from build123d import *

# Parameters (mm, degrees)
SKETCH1_R           = 4.7625
BOSS_EXTRUDE1_DEPTH = 0.79375
SKETCH2_R           = 3.9751
BOSS_EXTRUDE2_DEPTH = 5.461
SKETCH3_R           = 3.3147
BOSS_EXTRUDE3_DEPTH = 12.065
SKETCH6_R           = 1.5875
CUT_EXTRUDE1_DEPTH  = 19.05
SKETCH10_W          = 1.27
SKETCH10_H          = 1.778
SKETCH11_R          = 0.0508
CUT_EXTRUDE3_DEPTH  = 0.0254
SKETCH9_R           = 0.02
CUT_EXTRUDE2_DEPTH  = 23.4028
CHAMFER1_SIZE       = 1.27


with BuildPart() as part:
    # Sketch1 → Boss-Extrude1 (new body, symmetric)
    with BuildSketch(Plane.XY):
        Circle(SKETCH1_R)
    extrude(amount=BOSS_EXTRUDE1_DEPTH, both=True)

    # Sketch2 → Boss-Extrude2 (add)
    with BuildSketch(Plane(origin=(0, 0, -0.79375), x_dir=(-1, 0, 0), z_dir=(0, 0, -1))):
        with Locations(Location((0, 0, 0), (0, 0, 180))):  # turned: the seam where the file's is
            Circle(SKETCH2_R)
    extrude(amount=BOSS_EXTRUDE2_DEPTH)

    # Sketch3 → Boss-Extrude3 (add)
    with BuildSketch(Plane.XY.offset(0.79375)):
        Circle(SKETCH3_R)
    extrude(amount=BOSS_EXTRUDE3_DEPTH)

    # Sketch5 → Revolve1 (revolve)
    with BuildSketch(Plane(origin=(0, 0, 0), x_dir=(0, 0, -1), z_dir=(1, 0, 0)), mode=Mode.PRIVATE) as revolve1_sk:
        Polygon((-12.85875, 3.3147), (-16.17345, 0), (-12.85875, 0), align=None)
    revolve(revolve1_sk.sketch.rotate(Axis((0, 0, 0), (0, 0, 1)), 270), axis=Axis((0, 0, 0), (0, 0, 1)))  # turned: the seam where the file's is

    # Sketch6 → Cut-Extrude1 (cut)
    with BuildSketch(Plane(origin=(0, 0, -6.25475), x_dir=(-1, 0, 0), z_dir=(0, 0, -1))):
        Circle(SKETCH6_R)
    extrude(amount=-CUT_EXTRUDE1_DEPTH, mode=Mode.SUBTRACT)

    # Sketch10 → Cut-Revolve1 (revolve, cut)
    with BuildSketch(Plane(origin=(0, 0, 0), x_dir=(1, 0, 0), z_dir=(0, 1, 0)), mode=Mode.PRIVATE) as cut_revolve1_sk:
        with Locations((-3.3401, 1.68275)):
            Rectangle(SKETCH10_W, SKETCH10_H)
    revolve(cut_revolve1_sk.sketch.rotate(Axis((0, 0, 0), (0, 0, -1)), 180), axis=Axis((0, 0, 0), (0, 0, -1)), mode=Mode.SUBTRACT)  # turned: the seam where the file's is

    # Sketch11 → Cut-Extrude3 (cut)
    with BuildSketch(Plane.XY.offset(16.17345)):
        Circle(SKETCH11_R)
    extrude(amount=-CUT_EXTRUDE3_DEPTH, mode=Mode.SUBTRACT)

    # Sketch9 → Cut-Extrude2 (cut, through all)
    with BuildSketch(Plane(origin=(0, 0, -6.25475), x_dir=(-1, 0, 0), z_dir=(0, 0, -1))):
        Circle(SKETCH9_R)
    extrude(amount=-CUT_EXTRUDE2_DEPTH, mode=Mode.SUBTRACT)

    # Chamfer1
    chamfer1_edges = [part.edges().sort_by_distance(p)[0] for p in [
        (1.5875, 0, -6.25475),
    ]]
    chamfer(chamfer1_edges, length=CHAMFER1_SIZE)


solid = part.part
Could you check a few things on this model? Use its own coordinates, in mm. A direction names the side the tool comes from. Give positions to 0.01 mm unless a question says otherwise; leave off trailing zeros. Order: outer loops, then holes, each group sorted by start corner. A loop starts at its lowest first (then second) coordinate and runs counter-clockwise, first axis right, second up.
1. Suppose I cut it at D-D (z = 9). List the corners of the cut face in (x, y) for me (1 decimal).
2. Suppose I cut it at A-A (x = 3.75). List the corners of the cut face in (y, z) for me.
3. Suppose I cut it at C-C (y = 4.25). List the corners of the cut face in (x, z) for me, plus the area to 3 significant figures.
4. I need wall thicknesses on L1, parallel to Z at x = 3.5, y = 1.25; L2, parallel to Y at x = 0, z = 0; L3, parallel to Z at x = 3, y = 3. Which ranges of each line are inside material? Lowest first, please.
5. Suppose I cut it at B-B (z = -3.75). List the corners of the cut face in (x, y) for me (1 decimal).
6. For faces 5 (the flat face through (-0.3, 0, 12.795)), 6 (the cylindrical face through (-2.63, -2.02, 6.74)), 7 (the flat face through (3, 1, -2.572)), 8 (the cylindrical face through (-3.78, -2.9, 0.01)), which set-ups out of +Z, -Z, +X, -X, +Y, -Y let a thin tool reach every point of the face, with its end or its side?
7. Will these pins go through, and if not, where does the flat tip stop? P1, Ø4, axis at y = 2.5, z = 1.5, coming from the -X side; P2, Ø2, axis at y = 1.5, z = 5.5, coming from the +X side; P3, Ø1.9, axis at x = 0, y = 0, coming from the -Z side.
8. We'd pull the mould along Y, two halves only. Please class faces 1 (the cylindrical face through (2.58, -0.81, -1.7)), 2 (the cylindrical face through (0.34, -1.55, 3.78)), 3 (the flat face through (2, -3, 0.794)), 4 (the conical face through (-0.8, -1.5, -5.1)): pulls with the +Y half, pulls with the -Y half, needs draft (parallel to the pull), parting line crosses it, or undercut.
Solved:
1. outline: circle Ø6.6 at (0, 0); hole circle Ø3.2 at (0, 0)
2. outline: (-2.94, -0.79) - (2.94, -0.79) - (2.94, 0.79) - (-2.94, 0.79) - close; (-1.32, -6.25) - (1.32, -6.25) - (1.32, -2.57) - (-1.32, -2.57) - close
3. outline: (-2.15, -0.79) - (2.15, -0.79) - (2.15, 0.79) - (-2.15, 0.79) - close
3. area: 6.82 mm2
4. L1: z = -6.25 to -2.57, -0.79 to 0.79
4. L2: y = -4.76 to -1.59, 1.59 to 4.76
4. L3: z = -0.79 to 0.79
5. outline: circle Ø8 at (0, 0); hole circle Ø3.2 at (0, 0)
6. face 5: -Z
6. face 6: +Z
6. face 7: none
6. face 8: +Z, -Z
7. P1: stops at x = -4.72
7. P2: stops at x = 3.28
7. P3: stops at z = 12.8
8. face 1: parting line crosses it
8. face 2: undercut
8. face 3: needs draft
8. face 4: undercut
